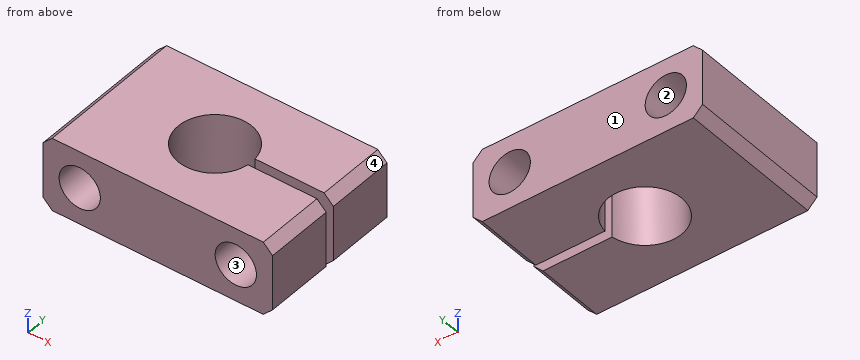
```python
from build123d import *

# Parameters (mm, degrees)
F0_W     = 25
F0_H     = 8
F0_R     = 2.25
F1_DEPTH = 16
F2_R     = 4
F3_DEPTH = 25
F4_SIZE  = 1
F6_DEPTH = 25


with BuildPart() as f1:
    # F0 (on Front) → F1 (new body)
    with BuildSketch(Plane.XZ):
        with Locations((10.216074, 3.959236)):
            Rectangle(F0_W, F0_H)
        with Locations((1.716074, 3.959236)):
            Circle(F0_R, mode=Mode.SUBTRACT)
        with Locations((18.716074, 3.959236)):
            Circle(F0_R, mode=Mode.SUBTRACT)
    extrude(amount=F1_DEPTH)

    # F2 (on face) → F3 (cut)
    with BuildSketch(Plane.XY.offset(7.959236)):
        with Locations((10.216074, -8)):
            Circle(F2_R)
    extrude(amount=-F3_DEPTH, mode=Mode.SUBTRACT)

    # F4
    f4_edges = [f1.edges().sort_by_distance(p)[0] for p in [
        (22.716074, -8, 7.959236),
        (22.716074, -8, -0.040764),
        (-2.283926, -8, 7.959236),
        (-2.283926, -8, -0.040764),
    ]]
    chamfer(f4_edges, length=F4_SIZE)

    # F5 (on face) → F6 (cut)
    with BuildSketch(Plane.XY.offset(7.959236)):
        with BuildLine():
            Line((22.760317, -7.5), (14.184701, -7.5))
            ThreePointArc((14.184701, -7.5), (14.216074, -8), (14.184701, -8.5))
            Line((14.184701, -8.5), (22.760317, -8.5))
            Line((22.760317, -8.5), (22.760317, -7.5))
        make_face()
    extrude(amount=-F6_DEPTH, mode=Mode.SUBTRACT)


solid = f1.part
```
Can you work these out from the model? Positions are in its coordinate system, mm. Face numbers are marked on the shaded views. Give positions to 0.01 mm unless a question says otherwise; leave off trailing zeros. Order: outer loops, then holes, each group sorted by start corner. A loop starts at its lowest first (then second) coordinate and runs counter-clockwise, first axis right, second up. Notation, with made-up numbers: (-16.75, -40) - (32.25, -40) arc R20 ccw to (32.25, -34) - close; hole circle Ø3 at (-32, 81.5). An arc over 180 degrees is marked (long way). Use a Markdown table: item, result. Add a question column.
Q1. If we section it at D-D on z = 4.5: Write out the boundary of the cut face in (x, y), plus the area to 3 significant figures.
Q2. Please list where these lines run through material, in increasing order: line 1 along Y through (x, z) = (17.5, 2); line 2 along X through (y, z) = (-6.5, 4); line 3 along X through (y, z) = (-11, 4).
Q3. I'm going to push a flat-ended pin straight in: pin 1 (2.5 mm diameter, centred on x = 16.5, z = 4.5, fed in from +Y). Where does the tip first touch, or does it pass through?
Q4. If we section it at C-C on x = 20.5: Write out the boundary of the cut face in (y, z).
Q5. If we mould it in two halves opening along X, with no side actions, what happens to the marked faces 1, 2, 3 and 4? For each: released by +X, released by -X, zero draft, split by the parting line, or undercut.
Q6. If we section it at B-B on y = -5: Write out the boundary of the cut face in (x, z), plus the area to 3 significant figures.
Q7. If we section it at A-A on x = 14.75: Write out the boundary of the cut face in (y, z).
Answers follow:
| question | item | result |
|---|---|---|
| 1 | outline | (-2.28, -16) - (-0.47, -16) - (-0.47, 0) - (-2.28, 0) - close; (3.9, -16) - (16.53, -16) - (16.53, -8.5) - (14.18, -8.5) arc R4 cw (long way) to (14.18, -7.5) - (16.53, -7.5) - (16.53, 0) - (3.9, 0) - close; (20.9, -16) - (22.72, -16) - (22.72, -8.5) - (20.9, -8.5) - close; (20.9, -7.5) - (22.72, -7.5) - (22.72, 0) - (20.9, 0) - close |
| 1 | area | 206 mm^2 |
| 2 | line 1 | y = -16 to -8.5, -7.5 to 0 |
| 2 | line 2 | x = -2.28 to -0.53, 3.97 to 6.51, 13.92 to 16.47, 20.97 to 22.72 |
| 2 | line 3 | x = -2.28 to -0.53, 3.97 to 7.57, 12.86 to 16.47, 20.97 to 22.72 |
| 3 | pin 1 | stops at y = 0 |
| 4 | outline | (-16, -0.04) - (-8.5, -0.04) - (-8.5, 2.59) - (-16, 2.59) - close; (-16, 5.33) - (-8.5, 5.33) - (-8.5, 7.96) - (-16, 7.96) - close; (-7.5, -0.04) - (0, -0.04) - (0, 2.59) - (-7.5, 2.59) - close; (-7.5, 5.33) - (0, 5.33) - (0, 7.96) - (-7.5, 7.96) - close |
| 5 | face 1 | zero draft |
| 5 | face 2 | undercut |
| 5 | face 3 | undercut |
| 5 | face 4 | released by +X |
| 6 | outline | (-2.28, 0.96) - (-1.28, -0.04) - (7.57, -0.04) - (7.57, 7.96) - (-1.28, 7.96) - (-2.28, 6.96) - close; (12.86, -0.04) - (21.72, -0.04) - (22.72, 0.96) - (22.72, 6.96) - (21.72, 7.96) - (12.86, 7.96) - close; hole circle Ø4.5 at (1.72, 3.96); hole circle Ø4.5 at (18.72, 3.96) |
| 6 | area | 124 mm^2 |
| 7 | outline | (-16, -0.04) - (-8.5, -0.04) - (-8.5, 7.96) - (-16, 7.96) - close; (-7.5, -0.04) - (0, -0.04) - (0, 7.96) - (-7.5, 7.96) - close |
